Job drawing, mm, ordinate dimensions from the low corner. One solid piece. Round coordinates to 2 decimals unless told otherwise and drop trailing zeros. Order: outer loops, then holes, each group sorted by start corner. A loop starts at its lowest first (then second) coordinate and runs counter-clockwise, first axis right, second up. Notation, with made-up numbers: (73, 84) -> (85, 84) arc R22 ccw to (85, 109) -> close; hole circle Ø11 at (81.25, -35). An arc over 180 degrees is marked (long way). Use CSV: the item, a comma, the result in double quotes.
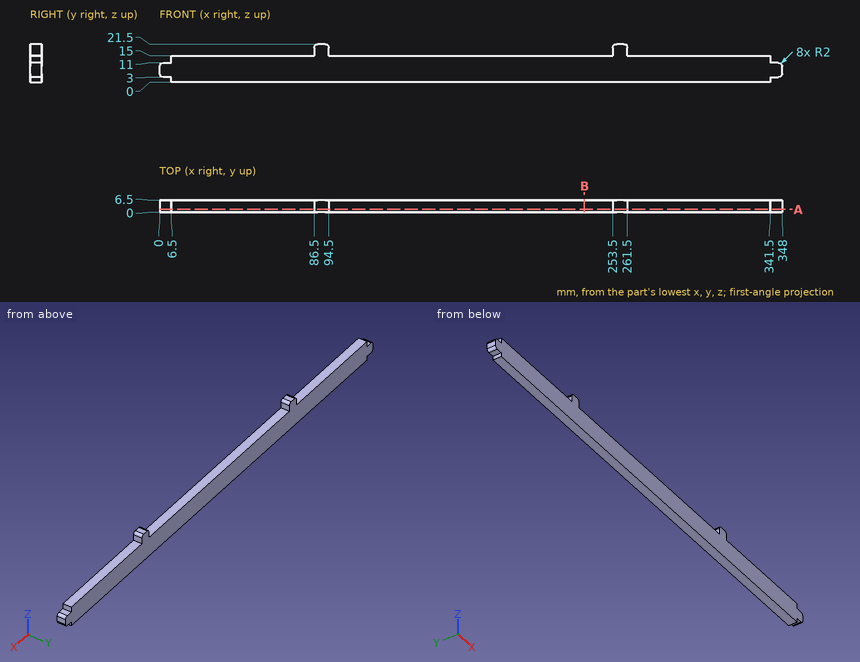
(1) Cut at A-A, the plane y = 1.5. Give the cut face in (x, z).
Reply:
outline,"(0, 5) arc R2 ccw to (2, 3) -> (6.5, 3) -> (6.5, 0) -> (341.5, 0) -> (341.5, 3) -> (346, 3) arc R2 ccw to (348, 5) -> (348, 9) arc R2 ccw to (346, 11) -> (341.5, 11) -> (341.5, 15) -> (261.5, 15) -> (261.5, 19.5) arc R2 ccw to (259.5, 21.5) -> (255.5, 21.5) arc R2 ccw to (253.5, 19.5) -> (253.5, 15) -> (94.5, 15) -> (94.5, 19.5) arc R2 ccw to (92.5, 21.5) -> (88.5, 21.5) arc R2 ccw to (86.5, 19.5) -> (86.5, 15) -> (6.5, 15) -> (6.5, 11) -> (2, 11) arc R2 ccw to (0, 9) -> close"
(2) Drop flat-ended pins along their axis: P1, Ø3.5, axis at x = 4.5, y = 2, coming from the -Z side; P2, Ø1.3, axis at y = 3.5, z = 18, coming from the -X side; P3, Ø2, axis at x = 3.5, y = 3.5, coming from the +Z side. Give the stop position or say it passes through.
Reply:
P1,"z = 3"
P2,"x = 86.5"
P3,"z = 11"
(3) Cut at B-B, the plane x = 237.5. Give the cut face in (y, z).
Reply:
outline,"(0, 0) -> (6.5, 0) -> (6.5, 15) -> (0, 15) -> close"
(4) Probe probe 1 along X at (y, z) = (1.75, 1.5); probe 2 along Z at (x, y) = (202, 6); probe 3 along X at (y, z) = (5.25, 4.5). List the from-to ranges inside material, lowest first. Write a range as [from, to].
Reply:
probe 1,"[6.5, 341.5]"
probe 2,"[0, 15]"
probe 3,"[0.06, 347.94]"
